Work out the finished part from the listing and answer in its coordinate system (mm). Coordinates: 2 decimals unless noted, no trailing zeros. Write each loop counter-clockwise with the first axis right and the second up, starting at its lowest first coordinate (ties: lowest second). Pieces come first, ordered by that corner, then holes. Notation, with made-up numbers: M 83,49 L 117,49 A16 ccw 117,55 Z; hole C 0,3 d11. An arc over 180 degrees is marked long. Answer as CSV lines item,"result". Start each with the question number.
(1) A cutting plane is placed at C-C on x = -418.75. Give the vertices of the cut face in (y, z), then the cut area to 4 significant figures.
(2) Flat-ended cylindrical pins translate along their axes: P1, Ø2.5, axis at x = -442.5, z = 3, coming from the -Y side; P2, Ø2.5, axis at y = -481.5, z = 2, coming from the +X side; P3, Ø2.5, axis at x = -419, z = 2.5, coming from the +Y side. Find the tip coordinate at first contact, or state that the pin passes through.
(3) A cutting plane is placed at A-A on y = -290.5. Give the vertices of the cut face in (x, z), then the cut area to 3 significant figures.
(4) A cutting plane is placed at D-D on y = -206. Give the vertices of the cut face in (x, z), then the cut area to 3 significant figures.
(5) Find the intervals of material crossed by L1, parallel to Y at x = -441.25, z = 3.05; L2, parallel to Y at x = -436.5, z = 4.1; L3, parallel to X at y = -185.5, z = 1.75, in increasing order. Write a range as [from, to].
from build123d import *

# Parameters (mm, degrees)
SKETCH1_W           = 5
SKETCH1_H           = 15
BOSS_EXTRUDE1_DEPTH = 5


with BuildPart() as part:
    # Sketch1 → Boss-Extrude1 (new body)
    with BuildSketch(Plane.XY):
        Polygon((-440, -217.5), (-440, -177.5), (-445, -177.5), (-445, -107.5), (-440, -107.5), (-440, -90), (-435, -90), (-435, -75), (-432.5, -75), (-432.5, -70), (-422.5, -70), (-422.5, -75), (-415, -75), (-415, -480), (-422.5, -480), (-422.5, -485), (-432.5, -485), (-432.5, -480), (-440, -480), (-440, -472.5), (-435, -472.5), (-435, -457.5), (-440, -457.5), (-440, -447.5), (-445, -447.5), (-445, -377.5), (-440, -377.5), (-440, -337.5), (-445, -337.5), (-445, -217.5), align=None)
        with Locations((-437.5, -291.25)):
            Rectangle(SKETCH1_W, SKETCH1_H, mode=Mode.SUBTRACT)
    extrude(amount=BOSS_EXTRUDE1_DEPTH)


solid = part.part
Here are the results:
1,outline,"M -480,0 L -75,0 L -75,5 L -480,5 Z"
1,area,"2,025 mm^2"
2,P1,"stops at y = -447.5"
2,P2,"stops at x = -422.5"
2,P3,"stops at y = -75"
3,outline,"M -445,0 L -440,0 L -440,5 L -445,5 Z; M -435,0 L -415,0 L -415,5 L -435,5 Z"
3,area,"125 mm^2"
4,outline,"M -440,0 L -415,0 L -415,5 L -440,5 Z"
4,area,"125 mm^2"
5,L1,"y = [-447.5, -377.5], [-337.5, -217.5], [-177.5, -107.5]"
5,L2,"y = [-480, -472.5], [-457.5, -298.75], [-283.75, -90]"
5,L3,"x = [-440, -415]"
